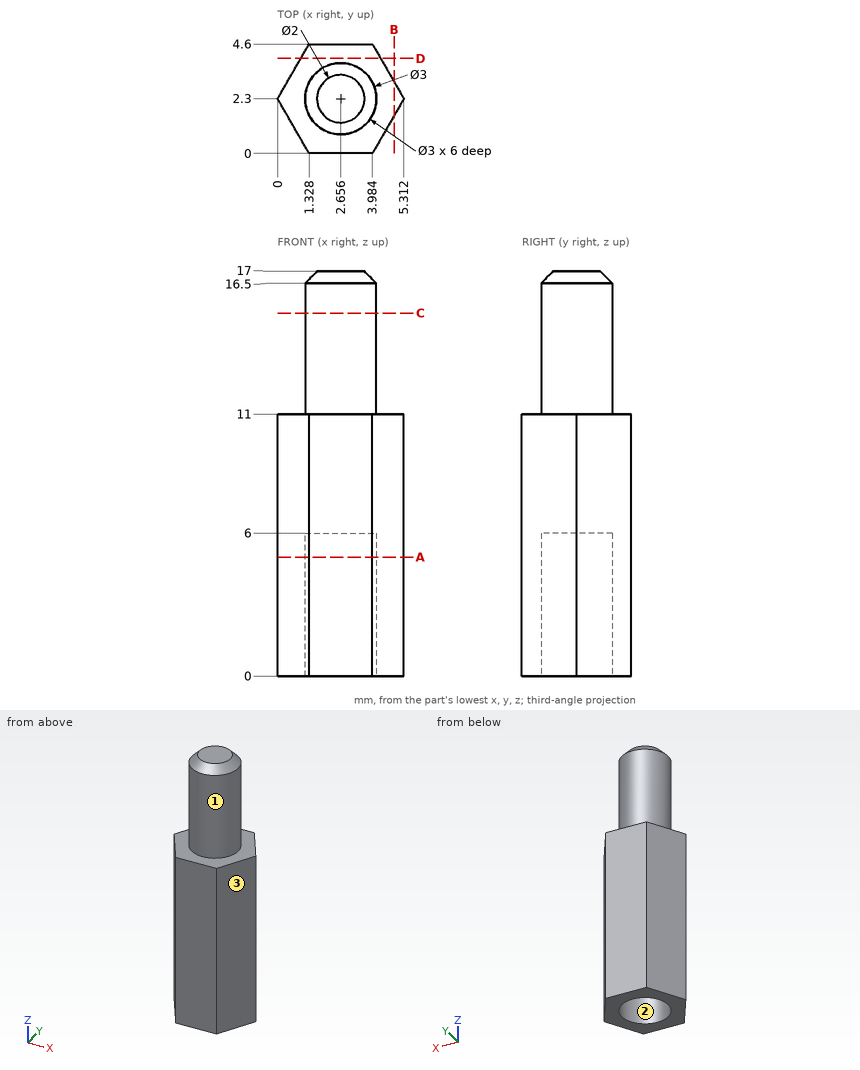
Can you work these out from the drawing? Everything is in mm from the part's minimum corner. Round coordinates to 2 decimals unless told otherwise and drop trailing zeros. Order: outer loops, then holes, each group sorted by start corner. A loop starts at its lowest first (then second) coordinate and runs counter-clockwise, first axis right, second up. Notation, with made-up numbers: M 24,9.25 L 66,9.25 A21 cw 66,40.25 Z; hole C 7,41 d6. An arc over 180 degrees is marked long. One line per question, with ' | ' between items.
1) I want a section at C-C, the plane z = 15.25. Write out the boundary of the cut face in (x, y) (1 decimal).
Working result:
outline: C 2.7,2.3 d3
2) I want a section at B-B, the plane x = 4.9. Write out the boundary of the cut face in (y, z), then the cut area to 3 significant figures.
Working result:
outline: M 1.59,0 L 3.01,0 L 3.01,11 L 1.59,11 Z | area: 15.7 mm²
3) If we mould it in two halves opening along Y, with no side actions, what happens to the marked faces 1, 2 and 3? For each: +Y half, -Y half, draft (parallel to the pull), parting line (faces both ways), or undercut.
Working result:
face 1: parting line | face 2: undercut | face 3: -Y half
4) I want a section at D-D, the plane y = 4. Write out the boundary of the cut face in (x, z).
Working result:
outline: M 0.98,0 L 4.33,0 L 4.33,11 L 0.98,11 Z
5) I want a section at A-A, the plane z = 5. Write out the boundary of the cut face in (x, y) (1 decimal).
Working result:
outline: M 0,2.3 L 1.3,0 L 4,0 L 5.3,2.3 L 4,4.6 L 1.3,4.6 Z; hole C 2.7,2.3 d3
6) For pin 1 Ø1 at (y, z) = (1.5, 5) entering from -X; pin 2 Ø1 at (x, z) = (3, 13.5) entering from -Y; pin 3 Ø0.9 at (x, y) = (2.5, 3) entering from -Z, each with a flat end and sliding along its axis, tell me the tip position at first contact or that it passes through.
Working result:
pin 1: x = 0.17 | pin 2: y = 0.8 | pin 3: z = 6
7) I need wall thicknesses on line 1 along X through (y, z) = (1.2, 1.25) (1 decimal); line 2 along Z through (x, y) = (3.05, 3.8); line 3 along Y through (x, z) = (3.5, 1.5). Which ranges of each line are inside material? Lowest first, please.
Working result:
line 1: 0.6 to 1.6, 3.7 to 4.7 | line 2: 0 to 11 | line 3: 0 to 1.06, 3.54 to 4.6
